from build123d import *

# Parameters (mm, degrees)
F0_W     = 18
F0_H     = 27
F1_DEPTH = 5
F2_SIZE  = 1
F3_R     = 4.75
F4_DEPTH = 1.5


with BuildPart() as f1:
    # F0 (on Top) → F1 (new body)
    with BuildSketch(Plane.XY):
        with Locations((13.321646, 17.421494)):
            Rectangle(F0_W, F0_H)
    extrude(amount=F1_DEPTH)

    # F2
    f2_edges = [f1.edges().sort_by_distance(p)[0] for p in [
        (4.321646, 30.921494, 2.5),
        (4.321646, 3.921494, 2.5),
        (22.321646, 3.921494, 2.5),
        (22.321646, 30.921494, 2.5),
        (22.321646, 17.421494, 0),
        (4.321646, 17.421494, 0),
        (13.321646, 3.921494, 0),
        (13.321646, 30.921494, 0),
    ]]
    chamfer(f2_edges, length=F2_SIZE)

    # F3 (on face) → F4 (cut)
    with BuildSketch(Plane.XY.offset(5)):
        with Locations((13.321646, 17.421494)):
            Circle(F3_R)
    extrude(amount=-F4_DEPTH, mode=Mode.SUBTRACT)


solid = f1.part
Input: part model. Units: mm. Frame: model coordinates. Coordinates: 2 decimals unless noted, no trailing zeros. Order: outer loops, then holes, each group sorted by start corner. A loop starts at its lowest first (then second) coordinate and runs counter-clockwise, first axis right, second up. Notation, with made-up numbers: M 73,38.25 L 129,38.25 A23 ccw 129,58.25 Z; hole C 0.25,14 d2. An arc over 180 degrees is marked long. Write item = value, one per line. Start each with the question number.
(1) Section A-A on z = 4.55. Output: boundary loops of the cut face in (x, y).
(2) First-contact query: P1, Ø3, axis at x = 12, y = 17.5, coming from the +Z side. Flat tip, straight axial feed; report the tip coordinate or a pass-through.
(3) Section C-C on y = 17. Output: boundary loops of the cut face in (x, z).
(4) Line query: line 1 along Z through (x, y) = (15.25, 15); line 2 along Y through (x, z) = (17.5, 4.3); line 3 along X through (y, z) = (21, 0.8). Output: solid intervals per line, ascending. Write a range as [from, to].
(5) Section B-B on x = 11. Output: boundary loops of the cut face in (y, z), and give its area (3 significant figures).
(6) Pull-direction query (X, two-part tool) for faces 1 (the flat face through (5, 30.2, 0.6)), 2 (the cylindrical face through (9.552, 14.531, 4.26)), 3 (the flat face through (13, 17, 3.5)), 4 (the flat face through (13, 18, 0)); classes: released by +X, released by -X, zero draft, split by the parting line, or undercut.
Result set:
q1.outline = M 4.32,4.92 L 5.32,3.92 L 21.32,3.92 L 22.32,4.92 L 22.32,29.92 L 21.32,30.92 L 5.32,30.92 L 4.32,29.92 Z; hole C 13.32,17.42 d9.5
q2.P1 = 3.5
q3.outline = M 4.32,1 L 5.32,0 L 21.32,0 L 22.32,1 L 22.32,5 L 18.05,5 L 18.05,3.5 L 8.59,3.5 L 8.59,5 L 4.32,5 Z
q4.line_1 = [0, 3.5]
q4.line_2 = [3.92, 15.16], [19.68, 30.92]
q4.line_3 = [4.52, 22.12]
q5.outline = M 3.92,1 L 4.92,0 L 29.92,0 L 30.92,1 L 30.92,5 L 21.57,5 L 21.57,3.5 L 13.28,3.5 L 13.28,5 L 3.92,5 Z
q5.area = 122 mm²
q6.face_1 = released by -X
q6.face_2 = undercut
q6.face_3 = undercut
q6.face_4 = zero draft
